Part model, mm, in its own coordinate system. Give positions to 0.01 mm unless a question says otherwise; leave off trailing zeros. Order: outer loops, then holes, each group sorted by start corner. A loop starts at its lowest first (then second) coordinate and runs counter-clockwise, first axis right, second up. Notation, with made-up numbers: (52, -4) -> (65, -4) arc R14 ccw to (65, 12) -> close; hole circle Ø8 at (-14.75, 85). An arc over 180 degrees is marked (long way). Write item = value, one per line. Start each with the question number.
Item 1: Drill centre lines: line 1 along Y through (x, z) = (-4, 1.1); line 2 along Y through (x, z) = (0, 1.15); line 3 along Y through (x, z) = (3.5, 1.35). Where is each one in solid material? Low to high.
Item 2: Band-saw the part on D-D on y = -22. Write the cut outline in (x, z).
Item 3: Band-saw the part on B-B on y = 22.5. Write the cut outline in (x, z).
Item 4: Band-saw the part on C-C on x = 5.5. Write the cut outline in (y, z).
Item 5: Flat gauge pin, fed straight in: P1, Ø2, axis at x = -1.33, y = 9, coming from the +Z side. Where does the tip first touch, or does it go through?
Item 6: Band-saw the part on A-A on z = 0.8. Count the separate pieces of the cut face and the enclosed holes in it, plus the area to 3 significant figures.
```python
from build123d import *

# Parameters (mm, degrees)
SKETCH1_W           = 16
SKETCH1_H           = 55
SKETCH1_R           = 1.5
BOSS_EXTRUDE1_DEPTH = 1.6
SKETCH3_R           = 0.65
CUT_EXTRUDE1_DEPTH  = 29.684664893
BOSS_EXTRUDE3_START = 0.05
SKETCH4_R           = 0.9
SKETCH4_R_2         = 0.65
SKETCH4_R_3         = 3.5
SKETCH4_R_4         = 1.5
SKETCH4_W           = 0.85
SKETCH4_H           = 3
SKETCH4_W_2         = 3
SKETCH4_H_2         = 4.8
BOSS_EXTRUDE3_DEPTH = 0.05


with BuildPart() as part:
    # Sketch1 → Boss-Extrude1 (new body)
    with BuildSketch(Plane.XY):
        Rectangle(SKETCH1_W, SKETCH1_H)
        with Locations((0, 22.5)):
            Circle(SKETCH1_R, mode=Mode.SUBTRACT)
    extrude(amount=BOSS_EXTRUDE1_DEPTH)

    # Sketch3 → Cut-Extrude1 (cut, through all)
    with BuildSketch(Plane.XY.offset(1.6)):
        with Locations((-4, -3.5)):
            Circle(SKETCH3_R)
        with Locations((-1.333333333, -3.5)):
            Circle(SKETCH3_R)
        with Locations((1.333333333, -3.5)):
            Circle(SKETCH3_R)
        with Locations((4, -3.5)):
            Circle(SKETCH3_R)
        with Locations((-4, 9)):
            Circle(SKETCH3_R)
        with Locations((-1.333333333, 9)):
            Circle(SKETCH3_R)
        with Locations((1.333333333, 9)):
            Circle(SKETCH3_R)
        with Locations((4, 9)):
            Circle(SKETCH3_R)
    extrude(amount=-CUT_EXTRUDE1_DEPTH, mode=Mode.SUBTRACT)

    # Sketch4 → Boss-Extrude3 (add)
    # profile 1 of 19: a face of its own
    with BuildSketch(Plane.XY.offset(1.6).offset(BOSS_EXTRUDE3_START)):
        with Locations(Location((-4, 9, 0), (0, 0, 180))):
            Circle(SKETCH4_R)
        with Locations((-4, 9)):
            Circle(SKETCH4_R_2, mode=Mode.SUBTRACT)
    # profile 2 of 19: a face of its own
    with BuildSketch(Plane.XY.offset(1.6).offset(BOSS_EXTRUDE3_START)):
        with Locations(Location((-1.333333333, 9, 0), (0, 0, 180))):
            Circle(SKETCH4_R)
        with Locations((-1.333333333, 9)):
            Circle(SKETCH4_R_2, mode=Mode.SUBTRACT)
    # profile 3 of 19: a face of its own
    with BuildSketch(Plane.XY.offset(1.6).offset(BOSS_EXTRUDE3_START)):
        with Locations(Location((1.333333333, 9, 0), (0, 0, 180))):
            Circle(SKETCH4_R)
        with Locations((1.333333333, 9)):
            Circle(SKETCH4_R_2, mode=Mode.SUBTRACT)
    # profile 4 of 19: a face of its own
    with BuildSketch(Plane.XY.offset(1.6).offset(BOSS_EXTRUDE3_START)):
        with Locations(Location((4, 9, 0), (0, 0, 180))):
            Circle(SKETCH4_R)
        with Locations((4, 9)):
            Circle(SKETCH4_R_2, mode=Mode.SUBTRACT)
    # profile 5 of 19: a face of its own
    with BuildSketch(Plane.XY.offset(1.6).offset(BOSS_EXTRUDE3_START)):
        with Locations(Location((4, -3.5, 0), (0, 0, 180))):
            Circle(SKETCH4_R)
        with Locations((4, -3.5)):
            Circle(SKETCH4_R_2, mode=Mode.SUBTRACT)
    # profile 6 of 19: a face of its own
    with BuildSketch(Plane.XY.offset(1.6).offset(BOSS_EXTRUDE3_START)):
        with Locations(Location((1.333333333, -3.5, 0), (0, 0, 180))):
            Circle(SKETCH4_R)
        with Locations((1.333333333, -3.5)):
            Circle(SKETCH4_R_2, mode=Mode.SUBTRACT)
    # profile 7 of 19: a face of its own
    with BuildSketch(Plane.XY.offset(1.6).offset(BOSS_EXTRUDE3_START)):
        with Locations(Location((-1.333333333, -3.5, 0), (0, 0, 180))):
            Circle(SKETCH4_R)
        with Locations((-1.333333333, -3.5)):
            Circle(SKETCH4_R_2, mode=Mode.SUBTRACT)
    # profile 8 of 19: a face of its own
    with BuildSketch(Plane.XY.offset(1.6).offset(BOSS_EXTRUDE3_START)):
        with Locations(Location((-4, -3.5, 0), (0, 0, 180))):
            Circle(SKETCH4_R)
        with Locations((-4, -3.5)):
            Circle(SKETCH4_R_2, mode=Mode.SUBTRACT)
    # profile 9 of 19: a face of its own
    with BuildSketch(Plane.XY.offset(1.6).offset(BOSS_EXTRUDE3_START)):
        with Locations(Location((0, 22.5, 0), (0, 0, 180))):
            Circle(SKETCH4_R_3)
        with Locations((0, 22.5)):
            Circle(SKETCH4_R_4, mode=Mode.SUBTRACT)
    # profile 10 of 19: a face of its own
    with BuildSketch(Plane.XY.offset(1.6).offset(BOSS_EXTRUDE3_START)):
        with Locations((-4.575, -8.5)):
            Rectangle(SKETCH4_W, SKETCH4_H)
    # profile 11 of 19: a face of its own
    with BuildSketch(Plane.XY.offset(1.6).offset(BOSS_EXTRUDE3_START)):
        with Locations((-3.267857143, -8.5)):
            Rectangle(SKETCH4_W, SKETCH4_H)
    # profile 12 of 19: a face of its own
    with BuildSketch(Plane.XY.offset(1.6).offset(BOSS_EXTRUDE3_START)):
        with Locations((-1.960714286, -8.5)):
            Rectangle(SKETCH4_W, SKETCH4_H)
    # profile 13 of 19: a face of its own
    with BuildSketch(Plane.XY.offset(1.6).offset(BOSS_EXTRUDE3_START)):
        with Locations((-0.653571429, -8.5)):
            Rectangle(SKETCH4_W, SKETCH4_H)
    # profile 14 of 19: a face of its own
    with BuildSketch(Plane.XY.offset(1.6).offset(BOSS_EXTRUDE3_START)):
        with Locations((0.653571429, -8.5)):
            Rectangle(SKETCH4_W, SKETCH4_H)
    # profile 15 of 19: a face of its own
    with BuildSketch(Plane.XY.offset(1.6).offset(BOSS_EXTRUDE3_START)):
        with Locations((1.960714286, -8.5)):
            Rectangle(SKETCH4_W, SKETCH4_H)
    # profile 16 of 19: a face of its own
    with BuildSketch(Plane.XY.offset(1.6).offset(BOSS_EXTRUDE3_START)):
        with Locations((3.267857143, -8.5)):
            Rectangle(SKETCH4_W, SKETCH4_H)
    # profile 17 of 19: a face of its own
    with BuildSketch(Plane.XY.offset(1.6).offset(BOSS_EXTRUDE3_START)):
        with Locations((4.575, -8.5)):
            Rectangle(SKETCH4_W, SKETCH4_H)
    # profile 18 of 19: a face of its own
    with BuildSketch(Plane.XY.offset(1.6).offset(BOSS_EXTRUDE3_START)):
        with Locations((-6, -21.1)):
            Rectangle(SKETCH4_W_2, SKETCH4_H_2)
    # profile 19 of 19: a face of its own
    with BuildSketch(Plane.XY.offset(1.6).offset(BOSS_EXTRUDE3_START)):
        with Locations((6, -21.1)):
            Rectangle(SKETCH4_W_2, SKETCH4_H_2)
    extrude(amount=-BOSS_EXTRUDE3_DEPTH)


solid = part.part
```
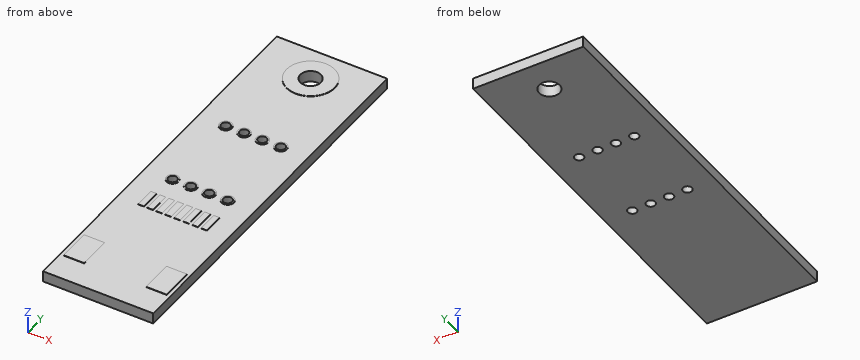
Values found:
q1.line_1 = -27.5 to -4.15, -2.85 to 8.35, 9.65 to 27.5
q1.line_2 = -27.5 to 21, 24 to 27.5
q1.line_3 = -27.5 to -3.92, -3.08 to 8.58, 9.42 to 27.5
q2.outline = (-8, 0) -> (8, 0) -> (8, 1.6) -> (7.5, 1.6) -> (7.5, 1.65) -> (4.5, 1.65) -> (4.5, 1.6) -> (-4.5, 1.6) -> (-4.5, 1.65) -> (-7.5, 1.65) -> (-7.5, 1.6) -> (-8, 1.6) -> close
q3.outline = (-8, 0) -> (-1.5, 0) -> (-1.5, 1.65) -> (-3.5, 1.65) -> (-3.5, 1.6) -> (-8, 1.6) -> close; (1.5, 0) -> (8, 0) -> (8, 1.6) -> (3.5, 1.6) -> (3.5, 1.65) -> (1.5, 1.65) -> close
q4.outline = (-27.5, 0) -> (27.5, 0) -> (27.5, 1.6) -> (-18.7, 1.6) -> (-18.7, 1.65) -> (-23.5, 1.65) -> (-23.5, 1.6) -> (-27.5, 1.6) -> close
q5.P1 = 1.65
q6.separate_pieces = 1
q6.enclosed_holes = 9
q6.area = 862 mm^2
